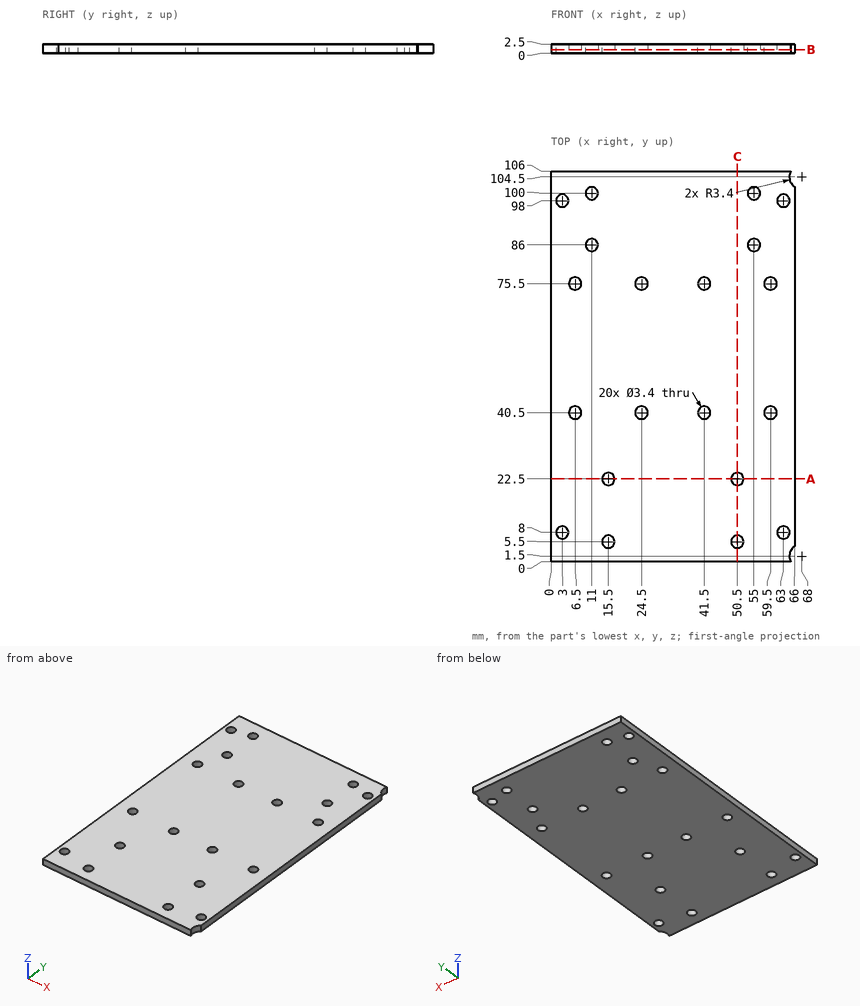
Print and shaded views of the part. All mm, measured from the part's lowest x, y and z. Coordinates: 2 decimals unless noted, no trailing zeros. Loops run counter-clockwise (first coordinate to the right, second up) from the corner with the lowest first, then second, coordinate; pieces in that order, holes last. Notation, with made-up numbers: (30.25, -1.5) -> (70.25, -1.5) arc R10 cw to (70.25, 2.5) -> close; hole circle Ø2 at (60.25, 89.5). An arc over 180 degrees is marked (long way). Use a Markdown table: item, result. Add a question column.
Item 1: Band-saw the part on B-B on z = 0.95. Give the number of separate pieces and of enclosed holes in the cut face, plus the area to 3 significant figures.
Item 2: Probe probe 1 along X at (y, z) = (86, 1.8); probe 2 along X at (y, z) = (75.5, 1.2); probe 3 along Y at (x, z) = (6.5, 1.55). List the from-to ranges inside material, lowest first.
Item 3: Flat gauge pins, fed straight in: P1, Ø2, axis at x = 6.5, y = 75.5, coming from the +Z side; P2, Ø4.5, axis at x = 63, y = 98, coming from the -Z side. Where does each tip first touch, or does it go through?
Item 4: Band-saw the part on C-C on x = 50.5. Write the cut outline in (y, z), plus the area to 3 significant figures.
Item 5: Band-saw the part on A-A on y = 22.5. Write the cut outline in (x, z).
Geometry says:
| question | item | result |
|---|---|---|
| 1 | separate pieces | 1 |
| 1 | enclosed holes | 20 |
| 1 | area | 6,810 mm² |
| 2 | probe 1 | 0 to 9.3, 12.7 to 53.3, 56.7 to 66 |
| 2 | probe 2 | 0 to 4.8, 8.2 to 22.8, 26.2 to 39.8, 43.2 to 57.8, 61.2 to 66 |
| 2 | probe 3 | 0 to 38.8, 42.2 to 73.8, 77.2 to 106 |
| 3 | P1 | through |
| 3 | P2 | z = 0 |
| 4 | outline | (0, 0) -> (3.8, 0) -> (3.8, 2.5) -> (0, 2.5) -> close; (7.2, 0) -> (20.8, 0) -> (20.8, 2.5) -> (7.2, 2.5) -> close; (24.2, 0) -> (106, 0) -> (106, 2.5) -> (24.2, 2.5) -> close |
| 4 | area | 248 mm² |
| 5 | outline | (0, 0) -> (13.8, 0) -> (13.8, 2.5) -> (0, 2.5) -> close; (17.2, 0) -> (48.8, 0) -> (48.8, 2.5) -> (17.2, 2.5) -> close; (52.2, 0) -> (66, 0) -> (66, 2.5) -> (52.2, 2.5) -> close |
